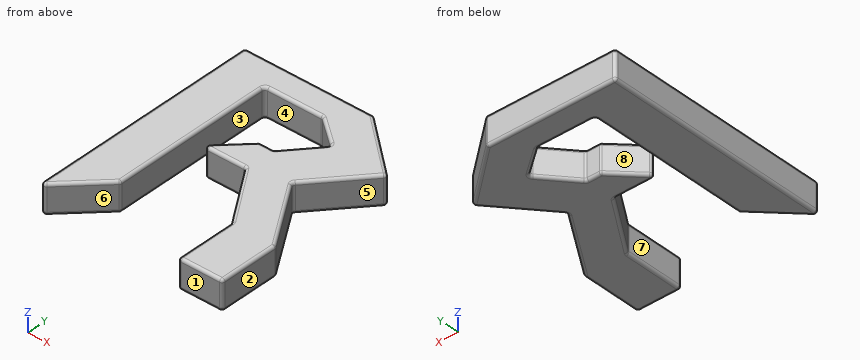
```python
from build123d import *

# Parameters (mm, degrees)
BOSS_EXTRUDE1_DEPTH = 10
FILLET3_R           = 1


with BuildPart() as part:
    # Sketch3 → Boss-Extrude1 (new body)
    with BuildSketch(Plane.XY):
        Polygon((0, 69.747073231), (0, 0), (0, -10), (15.06772633, 5.06772633), (15.06772633, 15.577629005), (15.06772633, 60.522611967), (34.746102146, 60.522611967), (44.75412708, 52.626214838), (35.220089692, 41.487878952), (30.220089692, 41.487878952), (19.613487974, 30.881277234), (34.746102146, 30.881277234), (48.208411003, 10.536544123), (48.208411003, 0), (48.208411003, -10), (63.3304478, -10), (63.3304478, -0.075498865), (63.3304478, 0), (63.3304478, 10.536544123), (48.208411003, 33.963716022), (64.182876427, 52.626214838), (44.18108037, 69.747073231), align=None)
    extrude(amount=BOSS_EXTRUDE1_DEPTH)

    # Fillet3
    fillet3_edges = [part.edges().sort_by_distance(p)[0] for p in [
        (48.208411003, 0.268272062, 10),
        (55.769429402, -10, 10),
        (27.17979506, 30.881277234, 0),
        (24.916788833, 36.184578093, 0),
        (32.720089692, 41.487878952, 0),
        (39.987108386, 47.057046895, 0),
        (39.750114613, 56.574413402, 0),
        (24.906914238, 60.522611967, 0),
        (63.3304478, 0.268272062, 10),
        (15.06772633, 32.795169148, 0),
        (7.533863165, -2.466136835, 0),
        (0, 29.873536616, 0),
        (22.090540185, 69.747073231, 0),
        (54.181978398, 61.186644035, 0),
        (56.195643715, 43.29496543, 0),
        (55.769429402, 22.250130073, 0),
        (63.3304478, 0.268272062, 0),
        (55.769429402, -10, 0),
        (48.208411003, 0.268272062, 0),
        (41.477256575, 20.708910679, 0),
        (55.769429402, 22.250130073, 10),
        (34.746102146, 30.881277234, 5),
        (19.613487974, 30.881277234, 5),
        (30.220089692, 41.487878952, 5),
        (35.220089692, 41.487878952, 5),
        (44.75412708, 52.626214838, 5),
        (56.195643715, 43.29496543, 10),
        (34.746102146, 60.522611967, 5),
        (15.06772633, 60.522611967, 5),
        (15.06772633, 5.06772633, 5),
        (0, -10, 5),
        (0, 69.747073231, 5),
        (44.18108037, 69.747073231, 5),
        (64.182876427, 52.626214838, 5),
        (48.208411003, 33.963716022, 5),
        (63.3304478, 10.536544123, 5),
        (63.3304478, -10, 5),
        (48.208411003, -10, 5),
        (48.208411003, 10.536544123, 5),
        (54.181978398, 61.186644035, 10),
        (22.090540185, 69.747073231, 10),
        (0, 29.873536616, 10),
        (7.533863165, -2.466136835, 10),
        (41.477256575, 20.708910679, 10),
        (15.06772633, 32.795169148, 10),
        (24.906914238, 60.522611967, 10),
        (39.750114613, 56.574413402, 10),
        (39.987108386, 47.057046895, 10),
        (32.720089692, 41.487878952, 10),
        (24.916788833, 36.184578093, 10),
        (27.17979506, 30.881277234, 10),
    ]]
    fillet(fillet3_edges, radius=FILLET3_R)


solid = part.part
```
Model file for the job. Use its own axes, mm. Face numbers are marked on the shaded views. A direction names the side the tool comes from. Give positions to 0.01 mm unless a question says otherwise; leave off trailing zeros. Use a Markdown table: item, result.
1) Pin check, flat tips, straight feed: pin 1 (3 mm diameter, centred on y = 9.5, z = 3.5, fed in from +X); pin 2 (4 mm diameter, centred on x = 26.5, z = 4.5, fed in from -Y); pin 3 (2.5 mm diameter, centred on y = 22, z = 3.5, fed in from +X). Stop position of each tip, or through.
Responses:
| item | result |
|---|---|
| pin 1 | stops at x = 63.33 |
| pin 2 | stops at y = 30.88 |
| pin 3 | stops at x = 56.74 |
2) Pull direction Y, two halves, no side cores. Call the marked faces 5, 6, 7 and 8: +Y half, -Y half, draft (parallel to the pull), parting line (faces both ways), or undercut.
Responses:
| item | result |
|---|---|
| face 5 | undercut |
| face 6 | -Y half |
| face 7 | draft |
| face 8 | undercut |
3) Drill centre lines: line 1 (X direction, y = 8.5, z = 6.75); line 2 (Y direction, x = 33.5, z = 6.5); line 3 (X direction, y = 36, z = 8). Where is each one in solid material? Low to high. Write a range as from..to.
Responses:
| item | result |
|---|---|
| line 1 | x = 0..15.07, 48.21..63.33 |
| line 2 | y = 30.88..41.49, 60.52..69.75 |
| line 3 | x = 0..15.07, 24.73..49.95 |
4) Tool access for the marked faces 1, 2, 3 and 4: list every direction of +Z, -Z, +X, -X, +Y, -Y with a clear straight run to the whole face (end or side of a thin tool).
Responses:
| item | result |
|---|---|
| face 1 | +Z, -Z, +X, -X, -Y |
| face 2 | +Z, -Z, +X, -Y |
| face 3 | +Z, -Z, -Y |
| face 4 | +Z, -Z |
